Input: dimensioned drawing with shaded views. Units: mm. Origin: part minimum x, y, z. A direction names the side the tool comes from. Coordinates: 2 decimals unless noted, no trailing zeros. Order: outer loops, then holes, each group sorted by start corner. A loop starts at its lowest first (then second) coordinate and runs counter-clockwise, first axis right, second up. Notation, with made-up numbers: (51.25, 81.25) -> (96.25, 81.25) arc R10 cw to (96.25, 97.25) -> close; hole circle Ø8 at (52.25, 72.5). An arc over 180 degrees is marked (long way). Put each result on its own line as item: value.
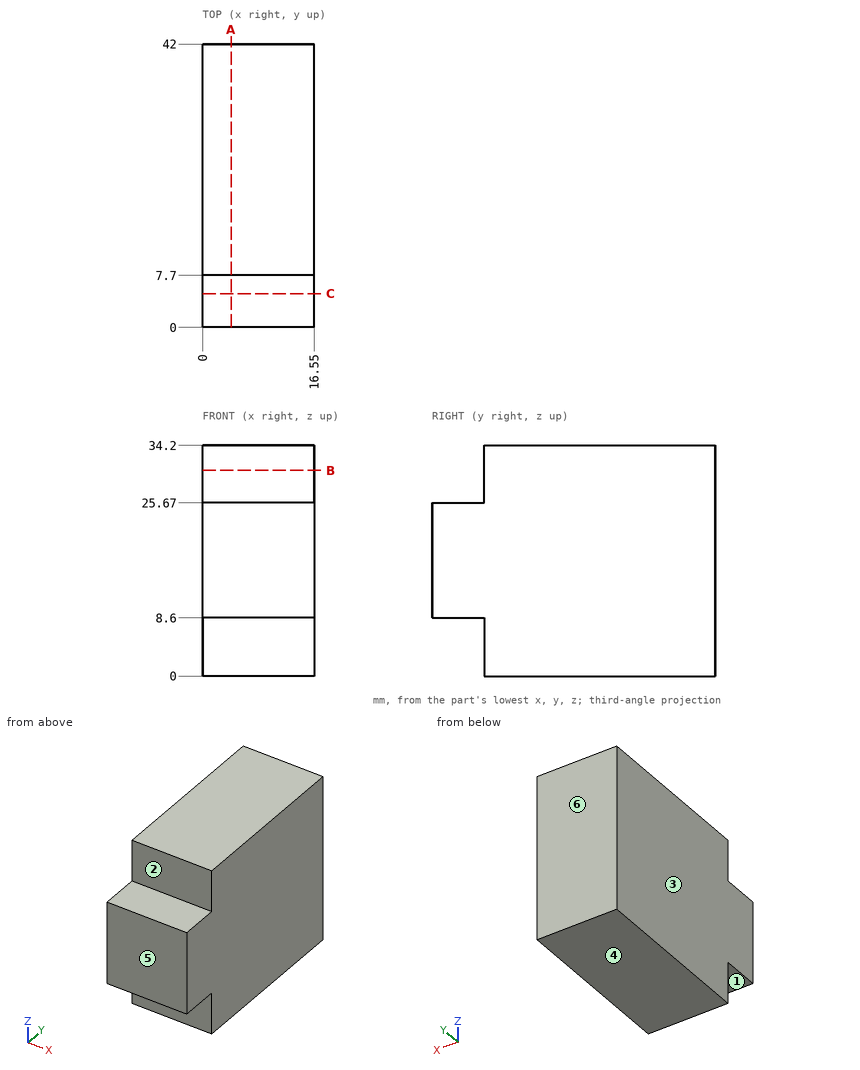
1. Cut plane C-C on y = 5. Output: boundary loops of the cut face in (x, z), plus the area to 3 significant figures.
Numbers:
outline: (0, 8.6) -> (16.55, 8.6) -> (16.55, 25.67) -> (0, 25.67) -> close
area: 283 mm2
2. Cut plane B-B on z = 30.5. Output: boundary loops of the cut face in (x, y), plus the area to 3 significant figures.
Numbers:
outline: (0, 7.7) -> (16.55, 7.7) -> (16.55, 42) -> (0, 42) -> close
area: 568 mm2
3. Ray query, line 1 along Y through (x, z) = (4.25, 7.5); line 2 along Z through (x, y) = (1, 2). Return the intervals inside material, ascending.
Numbers:
line 1: y = 7.7 to 42
line 2: z = 8.6 to 25.67
4. Pull-direction query (Y, two-part tool) for the marked faces 4, 5 and 6; classes: pulls with the +Y half, pulls with the -Y half, needs draft (parallel to the pull), parting line crosses it, or undercut.
Numbers:
face 4: needs draft
face 5: pulls with the -Y half
face 6: pulls with the +Y half
5. Set-up query: the marked faces 1, 2 and 3. Return all of +Z, -Z, +X, -X, +Y, -Y with unobstructed straight access to the full face (end or side cutting, diameter ignored); none if empty.
Numbers:
face 1: -Z, +X, -X, -Y
face 2: +Z, +X, -X, -Y
face 3: +Z, -Z, -X, +Y, -Y
6. First-contact query: pin 1 (4.5 mm diameter, centred on x = 11.5, z = 28.5, fed in from -Y); pin 2 (4 mm diameter, centred on x = 12, y = 4, fed in from +Z); pin 3 (3 mm diameter, centred on x = 8.5, y = 14.5, fed in from -Z); pin 4 (2.5 mm diameter, centred on x = 9.5, y = 4.5, fed in from -Z). Flat tips, straight axial feed; report the tip coordinate or a pass-through.
Numbers:
pin 1: stops at y = 7.7
pin 2: stops at z = 25.67
pin 3: stops at z = 0
pin 4: stops at z = 8.6
7. Cut plane A-A on x = 4.25. Output: boundary loops of the cut face in (y, z).
Numbers:
outline: (0, 8.6) -> (7.7, 8.6) -> (7.7, 0) -> (42, 0) -> (42, 34.2) -> (7.7, 34.2) -> (7.7, 25.67) -> (0, 25.67) -> close
